from build123d import *

# Parameters (mm, degrees)
F0_R     = 4
F1_DEPTH = 2.5
F2_R     = 5
F3_DEPTH = 50


with BuildPart() as f1:
    # F0 (on Top) → F1 (new body, symmetric)
    with BuildSketch(Plane.XY):
        with BuildLine():
            ThreePointArc((49.749372, -5), (49.937304, -2.503139), (50, 0))
            ThreePointArc((50, 0), (49.937304, 2.503139), (49.749372, 5))
            ThreePointArc((49.749372, 5), (35.355339, 35.355339), (5, 49.749372))
            ThreePointArc((5, 49.749372), (2.503139, 49.937304), (0, 50))
            ThreePointArc((0, 50), (-2.503139, 49.937304), (-5, 49.749372))
            ThreePointArc((-5, 49.749372), (-35.355339, 35.355339), (-49.749372, 5))
            ThreePointArc((-49.749372, 5), (-49.937304, 2.503139), (-50, 0))
            ThreePointArc((-50, 0), (-49.937304, -2.503139), (-49.749372, -5))
            ThreePointArc((-49.749372, -5), (-35.355339, -35.355339), (-5, -49.749372))
            ThreePointArc((-5, -49.749372), (-2.503139, -49.937304), (0, -50))
            ThreePointArc((0, -50), (2.503139, -49.937304), (5, -49.749372))
            ThreePointArc((5, -49.749372), (35.355339, -35.355339), (49.749372, -5))
        make_face()
        with BuildLine():
            ThreePointArc((-5, 55), (-3.535534, 51.464466), (0, 50))
            ThreePointArc((0, 50), (3.535534, 51.464466), (5, 55))
            ThreePointArc((5, 55), (0, 60), (-5, 55))
        make_face()
        with BuildLine():
            ThreePointArc((4, 55), (2.828427, 52.171573), (0, 51))
            ThreePointArc((0, 51), (-2.828427, 57.828427), (4, 55))
        make_face(mode=Mode.SUBTRACT)
        with BuildLine():
            ThreePointArc((-5, 49.749372), (-2.503139, 49.937304), (0, 50))
            ThreePointArc((0, 50), (-3.535534, 51.464466), (-5, 55))
            Line((-5, 55), (-5, 49.749372))
        make_face()
        with BuildLine():
            ThreePointArc((0, 50), (2.503139, 49.937304), (5, 49.749372))
            Line((5, 49.749372), (5, 55))
            ThreePointArc((5, 55), (3.535534, 51.464466), (0, 50))
        make_face()
        with BuildLine():
            ThreePointArc((55, 5), (51.464466, 3.535534), (50, 0))
            ThreePointArc((50, 0), (51.464466, -3.535534), (55, -5))
            ThreePointArc((55, -5), (58.535534, -3.535534), (60, 0))
            ThreePointArc((60, 0), (58.535534, 3.535534), (55, 5))
        make_face()
        with Locations((55, 0)):
            Circle(F0_R, mode=Mode.SUBTRACT)
        with BuildLine():
            ThreePointArc((55, -5), (51.464466, -3.535534), (50, 0))
            ThreePointArc((50, 0), (49.937304, -2.503139), (49.749372, -5))
            Line((49.749372, -5), (55, -5))
        make_face()
        with BuildLine():
            ThreePointArc((49.749372, 5), (49.937304, 2.503139), (50, 0))
            ThreePointArc((50, 0), (51.464466, 3.535534), (55, 5))
            Line((55, 5), (49.749372, 5))
        make_face()
        with BuildLine():
            Line((5, -55), (5, -49.749372))
            ThreePointArc((5, -49.749372), (2.503139, -49.937304), (0, -50))
            ThreePointArc((0, -50), (3.535534, -51.464466), (5, -55))
        make_face()
        with BuildLine():
            ThreePointArc((-5, -55), (-3.535534, -51.464466), (0, -50))
            ThreePointArc((0, -50), (-2.503139, -49.937304), (-5, -49.749372))
            Line((-5, -49.749372), (-5, -55))
        make_face()
        with BuildLine():
            ThreePointArc((5, -55), (3.535534, -51.464466), (0, -50))
            ThreePointArc((0, -50), (-3.535534, -51.464466), (-5, -55))
            ThreePointArc((-5, -55), (0, -60), (5, -55))
        make_face()
        with Locations((0, -55)):
            Circle(F0_R, mode=Mode.SUBTRACT)
        with BuildLine():
            ThreePointArc((-55, -5), (-51.464466, -3.535534), (-50, 0))
            ThreePointArc((-50, 0), (-51.464466, 3.535534), (-55, 5))
            ThreePointArc((-55, 5), (-60, 0), (-55, -5))
        make_face()
        with Locations((-55, 0)):
            Circle(F0_R, mode=Mode.SUBTRACT)
        with BuildLine():
            Line((-55, -5), (-49.749372, -5))
            ThreePointArc((-49.749372, -5), (-49.937304, -2.503139), (-50, 0))
            ThreePointArc((-50, 0), (-51.464466, -3.535534), (-55, -5))
        make_face()
        with BuildLine():
            ThreePointArc((-50, 0), (-49.937304, 2.503139), (-49.749372, 5))
            Line((-49.749372, 5), (-55, 5))
            ThreePointArc((-55, 5), (-51.464466, 3.535534), (-50, 0))
        make_face()
    extrude(amount=F1_DEPTH, both=True)

    # F2 (on face) → F3 (join)
    with BuildSketch(Plane.XY.offset(2.5)):
        Circle(F2_R)
    extrude(amount=F3_DEPTH)


solid = f1.part
Can you work these out from the model? Positions are in its coordinate system, mm. A direction names the side the tool comes from. Round coordinates to 2 decimals unless told otherwise and drop trailing zeros. Write each loop counter-clockwise with the first axis right and the second up, starting at its lowest first coordinate (ties: lowest second). Pieces come first, ordered by that corner, then holes. Notation, with made-up numbers: (49.25, -32.75) - (95.25, -32.75) arc R32 cw to (95.25, -6.75) - close; hole circle Ø5 at (46, -35). An arc over 180 degrees is marked (long way). Write each question's results on one line, items separated by ' | '. Start each with the question number.
1) Please list where these lines run through material, in increasing order: line 1 (X direction, y = 55, z = 0.85); line 2 (Z direction, x = 37, y = -11); line 3 (X direction, y = -1, z = 16).
2) Which directions (+Z, -Z, +X, -X, +Y, -Y) give clear straight access to the entire face, cutting with the end or side of a thin tool? Please do faces 1 (the cylindrical face through (-1.08, -4.88, 27.15)), 2 (the flat face through (-5, 52, 0)), 3 (the flat face through (-52, -5, 0)), 4 (the flat face through (52, 5, 0)).
3) We'd pull the mould along Y, two halves only. Please class faces 5 (the cylindrical face through (-60, 0, 0)), 6 (the flat face through (5, -52, 0)), 7 (the cylindrical face through (-0.867, -58.905, -0.035)): released by +Y, released by -Y, zero draft, split by the parting line, or undercut.
4) Suppose I cut it at A-A (z = 6.5). List the corners of the cut face in (x, y) for me.
5) For pin 1 Ø1.5 at (y, z) = (51.5, -0.5) entering from +X; pin 2 Ø4 at (x, y) = (8, -41.5) entering from +Z; pin 3 Ø1.5 at (x, z) = (51, 0.5) entering from +Y, each with a flat end and sliding along its axis, tell me the tip position at first contact or that it passes through.
6) Suppose I cut it at C-C (x = -27.5). List the corners of the cut face in (y, z) for me, and give its area (3 significant figures).
7) Suppose I cut it at B-B (y = 48). List the corners of the cut face in (x, z) for me, and give its area (3 significant figures).
Here are the results:
1) line 1: x = -5 to -4, 4 to 5 | line 2: z = -2.5 to 2.5 | line 3: x = -4.9 to 4.9
2) face 1: +Z | face 2: +Z, -Z, -X, +Y | face 3: +Z, -Z, -X, -Y | face 4: +Z, -Z, +X, +Y
3) face 5: split by the parting line | face 6: zero draft | face 7: undercut
4) outline: circle Ø10 at (0, 0)
5) pin 1: stops at x = 5 | pin 2: stops at z = 2.5 | pin 3: stops at y = 5
6) outline: (-41.76, -2.5) - (41.76, -2.5) - (41.76, 2.5) - (-41.76, 2.5) - close | area: 418 mm2
7) outline: (-14, -2.5) - (14, -2.5) - (14, 2.5) - (-14, 2.5) - close | area: 140 mm2
